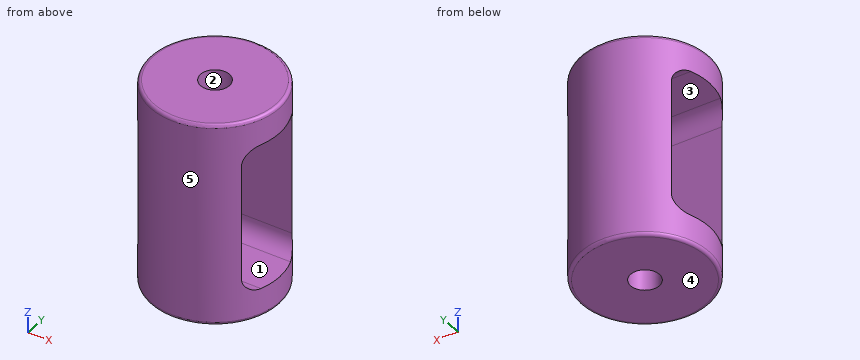
from build123d import *

# Parameters (mm, degrees)
BOSS_EXTRUDE1_DEPTH      = 16
BOSS_EXTRUDE1_DEPTH_BACK = 16
SKETCH1_R                = 10
SKETCH1_R_2              = 2.25
CUT_EXTRUDE1_DEPTH       = 22.354156504
CUT_EXTRUDE1_DEPTH_BACK  = 22.354156504
SKETCH2_W                = 23
SKETCH2_H                = 12
FILLET1_R                = 0.5
FILLET2_R                = 2.5


with BuildPart() as part:
    # Sketch1 → Boss-Extrude1 (new, two sides: drawn at the far end of the back side and taken through both)
    with BuildSketch(Plane.XY.offset(-BOSS_EXTRUDE1_DEPTH_BACK)):
        Circle(SKETCH1_R)
        Circle(SKETCH1_R_2, mode=Mode.SUBTRACT)
    extrude(amount=BOSS_EXTRUDE1_DEPTH + BOSS_EXTRUDE1_DEPTH_BACK)

    # Sketch2 → Cut-Extrude1 (cut, two sides: drawn at the far end of the back side and taken through both)
    with BuildSketch(Plane(origin=(0, 0, 0), x_dir=(0, 0, -1), z_dir=(1, 0, 0)).offset(-CUT_EXTRUDE1_DEPTH_BACK)):
        Rectangle(SKETCH2_W, SKETCH2_H)
    extrude(amount=CUT_EXTRUDE1_DEPTH + CUT_EXTRUDE1_DEPTH_BACK, mode=Mode.SUBTRACT)

    # Fillet1
    fillet1_edges = [part.edges().sort_by_distance(p)[0] for p in [
        (-10, 0, -16),
        (-10, 0, 16),
    ]]
    fillet(fillet1_edges, radius=FILLET1_R)

    # Fillet2
    fillet2_edges = [part.edges().sort_by_distance(p)[0] for p in [
        (0, -6, 11.5),
        (0, 6, -11.5),
        (0, 6, 11.5),
        (0, -6, -11.5),
    ]]
    fillet(fillet2_edges, radius=FILLET2_R)


solid = part.part
Here's how the part is built. I have some questions about the finished solid (model axes, mm). Face numbers are marked on the shaded views. A direction names the side the tool comes from. Coordinates: 2 decimals unless noted, no trailing zeros. Loops run counter-clockwise (first coordinate to the right, second up) from the corner with the lowest first, then second, coordinate; pieces in that order, holes last. Notation, with made-up numbers: (38, 38.5) -> (69, 38.5) arc R11 cw to (69, 50.5) -> close; hole circle Ø3 at (20.25, 85.25). An arc over 180 degrees is marked (long way). Use one line per item in the form item = value. Start each with the question number.
(1) Will these pins go through, and if not, where does the flat tip stop? pin 1 (2 mm diameter, centred on y = -3.5, z = -8, fed in from -X); pin 2 (1.5 mm diameter, centred on y = 5.5, z = -3.5, fed in from +X); pin 3 (1.5 mm diameter, centred on x = -4, z = -3.5, fed in from -Y); pin 4 (1 mm diameter, centred on x = 5.5, z = 10.5, fed in from -Y).
(2) We'd pull the mould along Y, two halves only. Please class the marked faces 3, 4 and 5: pulls with the +Y half, pulls with the -Y half, needs draft (parallel to the pull), parting line crosses it, or undercut.
(3) If we section it at B-B (x = 0): Please give me the cut outline in (y, z), then the cut area to 3 significant figures.
(4) Please list where these lines run through material, in increasing order: line 1 along Y through (x, z) = (0, 14); line 2 along Z through (x, y) = (-2.25, -3).
(5) If we section it at A-A (y = 0): Please give me the cut outline in (x, z), then the cut area to 3 significant figures.
(6) If we section it at D-D (z = -12): Please give me the cut outline in (x, y), then the cut area to 3 significant figures.
(7) On a 3-axis mill with a long thin cutter (end or side, diameter ignored), from which of +Z, -Z, +X, -X, +Y, -Y can I reach the whole of each face in a straight line? I mean the marked faces 1 and 2. Say none if no direction works.
(8) If we section it at C-C (z = 5): Please give me the cut outline in (x, y), then the cut area to 3 significant figures.
Verdict:
q1.pin_1 = through
q1.pin_2 = 8
q1.pin_3 = -9.46
q1.pin_4 = -8.66
q2.face_3 = undercut
q2.face_4 = needs draft
q2.face_5 = parting line crosses it
q3.outline = (-10, -15.5) arc R0.5 ccw to (-9.5, -16) -> (-2.25, -16) -> (-2.25, -11.5) -> (-3.5, -11.5) arc R2.5 cw to (-6, -9) -> (-6, 9) arc R2.5 cw to (-3.5, 11.5) -> (-2.25, 11.5) -> (-2.25, 16) -> (-9.5, 16) arc R0.5 ccw to (-10, 15.5) -> close; (2.25, -16) -> (9.5, -16) arc R0.5 ccw to (10, -15.5) -> (10, 15.5) arc R0.5 ccw to (9.5, 16) -> (2.25, 16) -> (2.25, 11.5) -> (3.5, 11.5) arc R2.5 cw to (6, 9) -> (6, -9) arc R2.5 cw to (3.5, -11.5) -> (2.25, -11.5) -> close
q3.area = 329 mm²
q4.line_1 = -10 to -2.25, 2.25 to 10
q4.line_2 = -16 to -11.5, 11.5 to 16
q5.outline = (-10, -15.5) arc R0.5 ccw to (-9.5, -16) -> (-2.25, -16) -> (-2.25, -11.5) -> (-10, -11.5) -> close; (-10, 11.5) -> (-2.25, 11.5) -> (-2.25, 16) -> (-9.5, 16) arc R0.5 ccw to (-10, 15.5) -> close; (2.25, -16) -> (9.5, -16) arc R0.5 ccw to (10, -15.5) -> (10, -11.5) -> (2.25, -11.5) -> close; (2.25, 11.5) -> (10, 11.5) -> (10, 15.5) arc R0.5 ccw to (9.5, 16) -> (2.25, 16) -> close
q5.area = 139 mm²
q6.outline = circle Ø20 at (0, 0); hole circle Ø4.5 at (0, 0)
q6.area = 298 mm²
q7.face_1 = +X, -X
q7.face_2 = +Z, -Z
q8.outline = (-8, -6) arc R10 ccw to (8, -6) -> close; (-8, 6) -> (8, 6) arc R10 ccw to start
q8.area = 89.5 mm²
